from build123d import *

# Parameters (mm, degrees)
SKETCH1_R           = 7.5
BOSS_EXTRUDE1_DEPTH = 60
SKETCH2_R           = 2
CUT_EXTRUDE1_DEPTH  = 5
CHAMFER1_SIZE       = 0.5
CUT_EXTRUDE2_START  = -5
SKETCH3_R           = 2
CUT_EXTRUDE2_DEPTH  = 5
CHAMFER2_SIZE       = 0.5


with BuildPart() as part:
    # Sketch1 → Boss-Extrude1 (new body)
    with BuildSketch(Plane(origin=(0, 0, 0), x_dir=(1, 0, 0), z_dir=(0, 1, 0))):
        with Locations(Location((0, 0, 0), (0, 0, 270))):
            Circle(SKETCH1_R)
    extrude(amount=BOSS_EXTRUDE1_DEPTH)

    # Sketch2 → Cut-Extrude1 (cut)
    with BuildSketch(Plane(origin=(0, 60, 0), x_dir=(1, 0, 0), z_dir=(0, 1, 0))):
        with Locations(Location((0, 0, 0), (0, 0, 270))):
            Circle(SKETCH2_R)
    extrude(amount=-CUT_EXTRUDE1_DEPTH, mode=Mode.SUBTRACT)

    # Chamfer1
    chamfer1_edges = [part.edges().sort_by_distance(p)[0] for p in [
        (0, 60, -2),
    ]]
    chamfer(chamfer1_edges, length=CHAMFER1_SIZE)

    # Sketch3 → Cut-Extrude2 (cut)
    with BuildSketch(Plane.XZ.offset(CUT_EXTRUDE2_START)):
        with Locations(Location((0, 0, 0), (0, 0, 90))):
            Circle(SKETCH3_R)
    extrude(amount=CUT_EXTRUDE2_DEPTH, mode=Mode.SUBTRACT)

    # Chamfer2
    chamfer2_edges = [part.edges().sort_by_distance(p)[0] for p in [
        (0, 0, -2),
    ]]
    chamfer(chamfer2_edges, length=CHAMFER2_SIZE)


solid = part.part
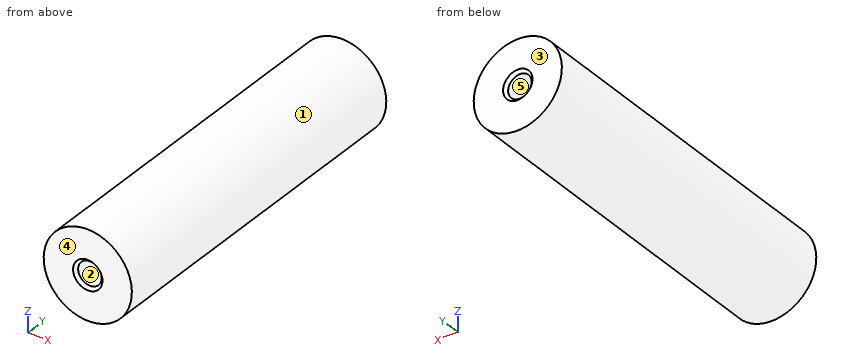
Geometry check sheet. Reference: the model listing, model coordinates, mm. Face numbers are marked on the shaded views. A direction names the side the tool comes from. Round coordinates to 2 decimals unless told otherwise and drop trailing zeros. Loops run counter-clockwise (first coordinate to the right, second up) from the corner with the lowest first, then second, coordinate; pieces in that order, holes last. Notation, with made-up numbers: (9, 0) - (28, 0) arc R13 cw to (28, 5) - close; hole circle Ø9 at (25, 65). An arc over 180 degrees is marked (long way). One line per question, with ' | ' between items. Start each with the question number.
1. Cross-section at A-A on x = 0. Record the cut outline in (y, z).
2. Cross-section at C-C on y = 25. Record the cut outline in (x, z).
3. Cross-section at B-B on z = 0. Record the cut outline in (x, y), then the cut area to 4 significant figures.
4. Cross-section at D-D on x = -6. Record the cut outline in (y, z).
5. Scan lines: line 1 (X direction, y = 3.25, z = 0); line 2 (Z direction, x = 3, y = 13); line 3 (Z direction, x = 1, y = 49.5). Record each from-to range of solid material in increasing order. Write a range as [from, to].
6. Tool access check on the marked faces 4 and 5. Record the directions out of +Z, -Z, +X, -X, +Y, -Y that give a thin tool (end or side, any length) a straight path to the whole face; none if there is none.
7. Depth check by flat-ended pin: pin 1 (1 mm diameter, centred on x = 3.5, y = 19.5, fed in from +Z); pin 2 (3 mm diameter, centred on x = 0, z = 0, fed in from +Y); pin 3 (4 mm diameter, centred on x = 3.5, y = 12, fed in from -Z). Enter the tip coordinate at first touch or a pass-through.
8. Draft check along Z on the marked faces 1, 2 and 3. Enter one of: released by +Z, released by -Z, zero draft, split by the parting line, or undercut.
Taken from the geometry:
1) outline: (0, -7.5) - (60, -7.5) - (60, -2.5) - (59.5, -2) - (55, -2) - (55, 2) - (59.5, 2) - (60, 2.5) - (60, 7.5) - (0, 7.5) - (0, 2.5) - (0.5, 2) - (5, 2) - (5, -2) - (0.5, -2) - (0, -2.5) - close
2) outline: circle Ø15 at (0, 0)
3) outline: (-7.5, 0) - (-2.5, 0) - (-2, 0.5) - (-2, 5) - (2, 5) - (2, 0.5) - (2.5, 0) - (7.5, 0) - (7.5, 60) - (2.5, 60) - (2, 59.5) - (2, 55) - (-2, 55) - (-2, 59.5) - (-2.5, 60) - (-7.5, 60) - close | area: 859.5 mm²
4) outline: (0, -4.5) - (60, -4.5) - (60, 4.5) - (0, 4.5) - close
5) line 1: [-7.5, -2], [2, 7.5] | line 2: [-6.87, 6.87] | line 3: [-7.43, 7.43]
6) face 4: +Z, -Z, +X, -X, -Y | face 5: +Y
7) pin 1: z = 6.87 | pin 2: y = 55 | pin 3: z = -7.35
8) face 1: split by the parting line | face 2: undercut | face 3: zero draft
